Check sheet for the modelled part. Datum: model origin and axes. Units: mm. Face numbers are marked on the shaded views. Round coordinates to 2 decimals unless told otherwise and drop trailing zeros. Write each loop counter-clockwise with the first axis right and the second up, starting at its lowest first coordinate (ties: lowest second). Pieces come first, ordered by that corner, then holes. Notation, with made-up numbers: M -35,82 L -19,82 A34 cw -19,119 Z; hole C 23,66 d9. An arc over 180 degrees is marked long. One line per item, written item: value.
from build123d import *

# Parameters (mm, degrees)
SKETCH_1_W             = 15
SKETCH_1_H             = 50
EXTRUDE_1_DEPTH        = 3
HOLE_WIZARD_M3_1_D     = 2.5
HOLE_WIZARD_M3_1_DEPTH = 3
HOLE_WIZARD_M3_1_2_D   = 3.4


with BuildPart() as part:
    # 스케치1 → 보스-돌출1 (new body)
    with BuildSketch(Plane.XY):
        Rectangle(SKETCH_1_W, SKETCH_1_H)
    extrude(amount=EXTRUDE_1_DEPTH)

    # Hole Wizard M3 _ _1
    with Locations(Plane.XY.offset(3)):
        with Locations((0, 5), (0, -5)):
            Hole(HOLE_WIZARD_M3_1_D / 2, depth=HOLE_WIZARD_M3_1_DEPTH)

    # Hole Wizard M3 _ _1 2 (through all)
    with Locations(Plane.XY.offset(3)):
        with Locations((-5, 22.5), (5, 22.5), (-5, -22.5), (5, -22.5)):
            Hole(HOLE_WIZARD_M3_1_2_D / 2)


solid = part.part
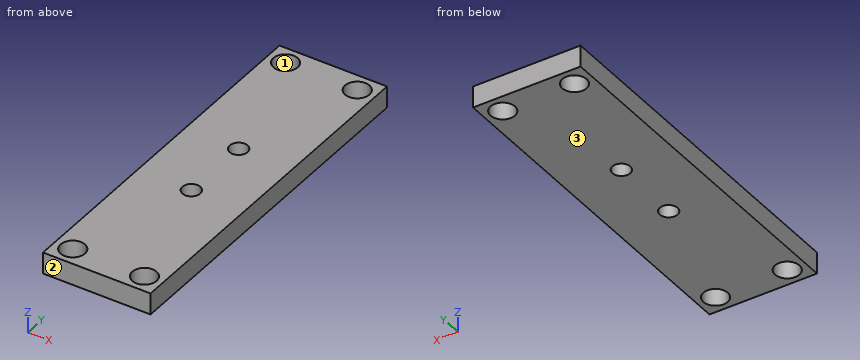
Q1. Scan lines: line 1 (Y direction, x = 0, z = 1.5); line 2 (Y direction, x = -5, z = 2.35). Record each from-to range of solid material in increasing order. Write a range as [from, to].
Completed:
line 1: [-25, -6.25], [-3.75, 3.75], [6.25, 25]
line 2: [-25, -24.2], [-20.8, 20.8], [24.2, 25]
Q2. Sectioned sample at B-B on y = 5. Enter the section's corners in (x, z), and give its area (3 significant figures).
Completed:
outline: M -7.5,0 L -1.25,0 L -1.25,3 L -7.5,3 Z; M 1.25,0 L 7.5,0 L 7.5,3 L 1.25,3 Z
area: 37.5 mm^2
Q3. Sectioned sample at A-A on x = 0. Enter the section's corners in (y, z).
Completed:
outline: M -25,0 L -6.25,0 L -6.25,3 L -25,3 Z; M -3.75,0 L 3.75,0 L 3.75,3 L -3.75,3 Z; M 6.25,0 L 25,0 L 25,3 L 6.25,3 Z
Q4. Depth check by flat-ended pin: P1, Ø2, axis at x = 5, y = -22.5, coming from the -Z side. Enter the tip coordinate at first touch or a pass-through.
Completed:
P1: through
Q5. Sectioned sample at C-C on z = 0.7. Enter the section's corners in (x, y), and give its area (3 significant figures).
Completed:
outline: M -7.5,-25 L 7.5,-25 L 7.5,25 L -7.5,25 Z; hole C -5,-22.5 d3.4; hole C -5,22.5 d3.4; hole C 0,-5 d2.5; hole C 0,5 d2.5; hole C 5,-22.5 d3.4; hole C 5,22.5 d3.4
area: 704 mm^2
Q6. Draft check along Y on the marked faces 1, 2 and 3. Enter one of: pulls with the +Y half, pulls with the -Y half, needs draft (parallel to the pull), parting line crosses it, or undercut.
Completed:
face 1: undercut
face 2: pulls with the -Y half
face 3: needs draft
Q7. Sectioned sample at D-D on x = -5. Enter the section's corners in (y, z).
Completed:
outline: M -25,0 L -24.2,0 L -24.2,3 L -25,3 Z; M -20.8,0 L 20.8,0 L 20.8,3 L -20.8,3 Z; M 24.2,0 L 25,0 L 25,3 L 24.2,3 Z
